from build123d import *

# Parameters (mm, degrees)
F1_DEPTH = 50.8
F3_DEPTH = 88.9


with BuildPart() as f1:
    # F0 (on Front) → F1 (new body, symmetric)
    with BuildSketch(Plane.XZ):
        Polygon((-19.63379, -40.465888), (-27.376695, -70.884436), (13.550079, -73.28105), (15.393632, -55.214275), (14.103146, -36.410082), (7.835083, -24.24266), (9.494272, -9.125564), (6.36024, 2.120081), (0, 8.756855), (29.588955, 20.924276), (31.432502, 26.270565), (26.454922, 29.404595), (20.555561, 26.086211), (-3.963629, 19.26508), (0, 25.34879), (18.343307, 35.488307), (22.767823, 41.940726), (19.633792, 48.577502), (8.203791, 45.812178), (11.153466, 48.577502), (14.139802, 56.377097), (10.784757, 61.113629), (-2.488789, 51.711533), (-15.209274, 30.695081), (-17.052822, 43.599918), (-12.509717, 65.082186), (-22.399113, 68.672173), (-32.169919, 41.756369), (-25.717501, 13.734437), (-30.695081, -6.175887), align=None)
    extrude(amount=F1_DEPTH, both=True)

    # F2 (on Right) → F3 (intersect, symmetric)
    with BuildSketch(Plane.YZ):
        Polygon((-28.482823, -58.163952), (-22.583468, -72.912343), (27.56105, -72.543629), (29.220244, -68.119116), (34.013465, -48.024435), (34.013465, -34.382179), (35.857018, -18.896371), (38.069274, -5.438467), (38.069274, 10.600403), (42.862501, 25.901856), (38.991049, 30.879436), (32.169919, 27.929757), (26.396504, 15.489846), (23.505243, 13.734437), (20.37121, 18.896371), (22.823287, 38.655246), (24.980079, 47.10266), (16.315402, 49.314924), (10.416048, 43.231212), (6.196184, 18.644363), (3.963629, 17.974596), (1.751371, 25.34879), (1.751371, 52.264594), (0, 65.722503), (-4.332338, 68.487823), (-7.282016, 65.538146), (-9.125565, 53.555083), (-9.125565, 25.717501), (-12.443951, 14.471854), (-14.471856, 27.376693), (-16.131047, 42.678144), (-16.131047, 60.744923), (-19.449435, 66.459917), (-25.717501, 64.985082), (-27.376695, 58.348306), (-29.588953, 43.599918), (-29.588953, 22.399114), (-26.086209, 4.885403), (-23.320887, -11.522178), (-28.298467, -27.745403), (-36.041372, -18.712016), (-38.622338, 0), (-43.784276, 4.147984), (-48.208792, 2.304435), (-48.208792, -3.041855), (-50.789759, -11.522178), (-40.834598, -36.594436), align=None)
    extrude(amount=F3_DEPTH, both=True, mode=Mode.INTERSECT)


solid = f1.part
Read the model definition and answer for the solid it produces. Units are mm, in the model's axes. A direction names the side the tool comes from. Round coordinates to 2 decimals unless told otherwise and drop trailing zeros. Loops run counter-clockwise (first coordinate to the right, second up) from the corner with the lowest first, then second, coordinate; pieces in that order, holes last.
Q1. Which of the six approach directions +Z, -Z, +X, -X, +Y, -Y give full straight-line access (tool end or side, diameter ignored) to faces 4 (the face through (-27.28, 35.2, 20.52)), 5 (the face through (9.043, -3.818, 30.348)), 6 (the face through (-4, 1.751, 39)), 7 (the face through (-3, 34.013, -41)), 8 (the face through (20.525, 16.273, 38.669))?
Q2. Consider probe 1 along Y at (x, z) = (-4, 30.5); probe 2 along Y at (x, z) = (-3.5, 21); probe 3 along Y at (x, z) = (-20, 46). Determine where each line is inside the solid, lowest interval first.
Q3. Determine the mould class of faces 1 (the face through (-19.293, -22.54, 65.733)), 2 (the face through (-20.09, -8.19, 59.63)), 3 (the face through (23.55, -3.76, 27.77)) for opening direction Y: released by +Y, released by -Y, zero draft, split by the parting line, or undercut.
Q4. Each of these flat-tipped pins is pushed along its axis until it touches: pin 1 (7 mm diameter, centred on x = 1.5, z = -39.5, fed in from +Y); pin 2 (8 mm diameter, centred on y = -39, z = -8, fed in from -X); pin 3 (22.5 mm diameter, centred on x = -12, z = 39, fed in from -Y). Where does it stop, or does it pass through?
Q5. Section A-A on z = 33.5 is taken. Write down the section's boundary in (x, y).
Output:
1. face 4: -X, +Y, -Y
1. face 5: +Y, -Y
1. face 6: +Z, +X, -X
1. face 7: -Z, +X, -X, +Y
1. face 8: +X, +Y, -Y
2. probe 1: y = -29.59 to -14.81, -9.13 to 1.75, 8.23 to 21.81, 38.11 to 39.29
2. probe 2: y = -29.31 to -13.47, -10.52 to 3.06, 6.6 to 20.63, 28.95 to 41.33
2. probe 3: y = -29.23 to -16.13, -9.13 to 1.75, 13.1 to 24.7
3. face 1: released by -Y
3. face 2: undercut
3. face 3: zero draft
4. pin 1: stops at y = 34.01
4. pin 2: stops at x = -30.7
4. pin 3: stops at y = -29.59
5. outline: (-30.27, -29.59) - (-15.61, -29.59) - (-15.61, -15.14) - (-30.27, -15.14) - close; (-30.27, -9.13) - (-15.61, -9.13) - (-15.61, 1.75) - (-30.27, 1.75) - close; (-30.27, 8.75) - (-15.61, 8.75) - (-15.61, 22.18) - (-30.27, 22.18) - close; (-13.51, -29.59) - (14.75, -29.59) - (14.75, -15.14) - (-13.51, -15.14) - close; (-13.51, -9.13) - (14.75, -9.13) - (14.75, 1.75) - (-13.51, 1.75) - close; (-13.51, 8.75) - (14.75, 8.75) - (14.75, 22.18) - (-13.51, 22.18) - close
